from build123d import *

# Parameters (mm, degrees)
SKETCH1_W           = 90.17
SKETCH1_H           = 60.77
BOSS_EXTRUDE1_DEPTH = 3.175
SKETCH2_W           = 30.83
SKETCH2_H           = 22.08
SKETCH2_W_2         = 31.83
CUT_EXTRUDE1_DEPTH  = 4.175
BOSS_EXTRUDE2_DEPTH = 3.175
FILLET1_R           = 5
SKETCH5_R           = 1.415
CUT_EXTRUDE2_DEPTH  = 10


with BuildPart() as part:
    # Sketch1 → Boss-Extrude1 (new body)
    with BuildSketch(Plane.XY):
        Rectangle(SKETCH1_W, SKETCH1_H)
    extrude(amount=BOSS_EXTRUDE1_DEPTH)

    # Sketch2 → Cut-Extrude1 (cut, through all)
    with BuildSketch(Plane.XY.offset(3.175)):
        with Locations((20.25, 14.675)):
            Rectangle(SKETCH2_W, SKETCH2_H)
        with Locations((-20.25, 14.675)):
            Rectangle(SKETCH2_W, SKETCH2_H)
        with Locations((0, -14.675)):
            Rectangle(SKETCH2_W_2, SKETCH2_H)
    extrude(amount=-CUT_EXTRUDE1_DEPTH, mode=Mode.SUBTRACT)

    # Sketch3 → Boss-Extrude2 (add)
    with BuildSketch(Plane.XY.offset(3.175)):
        with BuildLine():
            Line((45.085, 10.085), (45.085, -10.085))
            Line((45.085, -10.085), (75.085, -10.085))
            ThreePointArc((75.085, -10.085), (85.17, 0), (75.085, 10.085))
            Line((75.085, 10.085), (45.085, 10.085))
        make_face()
    extrude(amount=-BOSS_EXTRUDE2_DEPTH)

    # Fillet1
    fillet1_edges = [part.edges().sort_by_distance(p)[0] for p in [
        (45.085, -10.085, 1.5875),
        (45.085, 10.085, 1.5875),
    ]]
    fillet(fillet1_edges, radius=FILLET1_R)

    # Sketch5 → Cut-Extrude2 (cut)
    with BuildSketch(Plane.XY.offset(3.175)):
        with Locations((73.735, 0)):
            Circle(SKETCH5_R)
    extrude(amount=-CUT_EXTRUDE2_DEPTH, mode=Mode.SUBTRACT)


solid = part.part
Geometry check sheet. Reference: the model listing, model coordinates, mm. A direction names the side the tool comes from. Round coordinates to 2 decimals unless told otherwise and drop trailing zeros. Write each loop counter-clockwise with the first axis right and the second up, starting at its lowest first coordinate (ties: lowest second). Pieces come first, ordered by that corner, then holes.
Item 1: Material ranges on line 1 along X through (y, z) = (17.5, 2.3) (3 decimals); line 2 along Y through (x, z) = (-8, 2.15) (3 decimals); line 3 along Y through (x, z) = (17.5, 0.65) (3 decimals), recorded low to high.
Determined:
line 1: x = -45.085 to -35.665, -4.835 to 4.835, 35.665 to 45.085
line 2: y = -30.385 to -25.715, -3.635 to 3.635, 25.715 to 30.385
line 3: y = -30.385 to 3.635, 25.715 to 30.385
Item 2: Section check B-B (x = 0). Record the boundary of the cut face in (y, z) (3 decimals), plus the area to 3 significant figures.
Determined:
outline: (-30.385, 0) - (-25.715, 0) - (-25.715, 3.175) - (-30.385, 3.175) - close; (-3.635, 0) - (30.385, 0) - (30.385, 3.175) - (-3.635, 3.175) - close
area: 123 mm2
Item 3: Go/stop test with flat-tipped pins: pin 1 Ø1 at (x, z) = (60.5, 1.5) entering from +Y (3 decimals); pin 2 Ø1.6 at (x, z) = (62, 2) entering from -Y (3 decimals). Record where each tip stops, or that it passes through.
Determined:
pin 1: stops at y = 10.085
pin 2: stops at y = -10.085
Item 4: Section check D-D (y = -20). Record the boundary of the cut face in (x, z) (3 decimals).
Determined:
outline: (-45.085, 0) - (-15.915, 0) - (-15.915, 3.175) - (-45.085, 3.175) - close; (15.915, 0) - (45.085, 0) - (45.085, 3.175) - (15.915, 3.175) - close
Item 5: Section check C-C (y = 17.5). Record the boundary of the cut face in (x, z) (3 decimals), plus the area to 3 significant figures.
Determined:
outline: (-45.085, 0) - (-35.665, 0) - (-35.665, 3.175) - (-45.085, 3.175) - close; (-4.835, 0) - (4.835, 0) - (4.835, 3.175) - (-4.835, 3.175) - close; (35.665, 0) - (45.085, 0) - (45.085, 3.175) - (35.665, 3.175) - close
area: 90.5 mm2
Item 6: Section check A-A (z = 0.55). Record the boundary of the cut face in (x, y) (3 decimals), plus the area to 3 significant figures.
Determined:
outline: (-45.085, -30.385) - (45.085, -30.385) - (45.085, -15.085) arc R5 cw to (50.085, -10.085) - (75.085, -10.085) arc R10.085 ccw to (75.085, 10.085) - (50.085, 10.085) arc R5 cw to (45.085, 15.085) - (45.085, 30.385) - (-45.085, 30.385) - close; hole (-35.665, 3.635) - (-4.835, 3.635) - (-4.835, 25.715) - (-35.665, 25.715) - close; hole (-15.915, -25.715) - (15.915, -25.715) - (15.915, -3.635) - (-15.915, -3.635) - close; hole (4.835, 3.635) - (35.665, 3.635) - (35.665, 25.715) - (4.835, 25.715) - close; hole circle Ø2.83 at (73.735, 0)
area: 4,180 mm2
Item 7: Mould release check, pull along Y, two halves, no side actions. Record for faces 4 (the face through (45.085, 23, 2)), 5 (the face through (20, 3.635, 2)), 6 (the face through (46.5, -11.6, 1.6)): +Y half, -Y half, draft (parallel to the pull), parting line (faces both ways), or undercut.
Determined:
face 4: draft
face 5: undercut
face 6: -Y half
Item 8: Access from +Z, -Z, +X, -X, +Y, -Y to the whole of each face (thin tool, end or side, straight path). Record for faces 1 (the face through (5, 0, 0)), 2 (the face through (-15.915, -15, 2)), 3 (the face through (45.085, -23, 2)).
Determined:
face 1: -Z, +X, -X, +Y, -Y
face 2: +Z, -Z
face 3: +Z, -Z, +X, -Y
